The model under review builds one solid part; all positions refer to its coordinate system, in mm. Face numbers are marked on the shaded views. A direction names the side the tool comes from. Coordinates: 2 decimals unless noted, no trailing zeros. Order: outer loops, then holes, each group sorted by start corner. A loop starts at its lowest first (then second) coordinate and runs counter-clockwise, first axis right, second up. Notation, with made-up numbers: (84.5, -30) - (140.5, -30) arc R19 cw to (140.5, -9) - close; hole circle Ø2 at (-29, -39.5). An arc over 180 degrees is marked (long way). Answer in a Markdown table with one row per item.
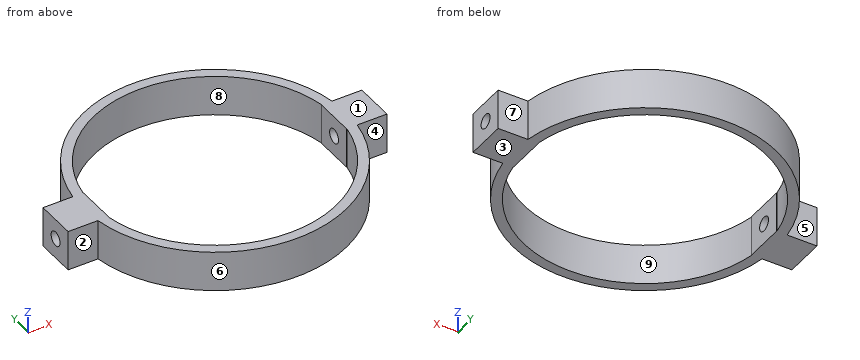
```python
from build123d import *

# Parameters (mm, degrees)
F0_R     = 41.275
F0_R_2   = 38.1
F1_DEPTH = 12.7
F3_W     = 12.7
F3_H     = 12.7
F4_DEPTH = 12.7
F6_W     = 12.7
F6_H     = 12.7
F7_DEPTH = 12.7
F9_D     = 4.4958


with BuildPart() as f1:
    # F0 (on Top) → F1 (new body)
    with BuildSketch(Plane.XY):
        Circle(F0_R)
        Circle(F0_R_2, mode=Mode.SUBTRACT)
    extrude(amount=F1_DEPTH)

    # F3 (on offset) → F4 (join)
    with BuildSketch(Plane.YZ.offset(37.465)):
        with Locations((0, 6.35)):
            Rectangle(F3_W, F3_H)
    extrude(amount=F4_DEPTH)

    # F6 (on offset) → F7 (join)
    with BuildSketch(Plane.YZ.offset(-37.465)):
        with Locations((0, 6.35)):
            Rectangle(F6_W, F6_H)
    extrude(amount=-F7_DEPTH)

    # F9 (through all)
    with Locations(Plane(origin=(-50.165, 0, 0), x_dir=(0, -1, 0), z_dir=(-1, 0, 0))):
        with Locations((0, 6.35)):
            Hole(F9_D / 2)


solid = f1.part
```
Item 1: Tool access review of the marked faces 1, 2, 3, 4 and 5: name each direction out of +Z, -Z, +X, -X, +Y, -Y from which nothing blocks a thin tool from reaching the whole face with its end or side.
Check values:
| item | result |
|---|---|
| face 1 | +Z, +X, -X, +Y, -Y |
| face 2 | +Z, -Z, -X, -Y |
| face 3 | -Z, +X, -X, +Y, -Y |
| face 4 | +Z, -Z, +X, -Y |
| face 5 | +Z, -Z, -X, +Y |
Item 2: We need section C-C, the plane x = 42. Write out the cut boundary in (y, z), then the cut area to 3 significant figures.
Check values:
| item | result |
|---|---|
| outline | (-6.35, 0) - (6.35, 0) - (6.35, 12.7) - (-6.35, 12.7) - close; hole circle Ø4.5 at (0, 6.35) |
| area | 145 mm^2 |
Item 3: To check wall thickness, follow line 1 (Z direction, x = 40.5, y = 0); line 2 (X direction, y = 5.5, z = 3) (3 decimals); line 3 (X direction, y = -32.5, z = 1.5). State the ranges of each line that lie inside material, in increasing order. Write a range as from..to.
Check values:
| item | result |
|---|---|
| line 1 | 0..4.1, 8.6..12.7 |
| line 2 | -50.165..-37.465, 37.465..50.165 |
| line 3 | -25.44..-19.88, 19.88..25.44 |
Item 4: We need section D-D, the plane y = 22. Write out the cut boundary in (x, z).
Check values:
| item | result |
|---|---|
| outline | (-34.92, 0) - (-31.11, 0) - (-31.11, 12.7) - (-34.92, 12.7) - close; (31.11, 0) - (34.92, 0) - (34.92, 12.7) - (31.11, 12.7) - close |
Item 5: Clearance check with flat-ended pins moving along their axes: pin 1 Ø4.5 at (x, z) = (45.5, 4.5) entering from +Y; pin 2 Ø2 at (x, z) = (-30, 4.5) entering from -Y; pin 3 Ø4.5 at (x, z) = (-45, 3) entering from -Y; pin 4 Ø2.5 at (y, z) = (0, 6.35) entering from -X. State where each tip first meets the part, or that it passes through.
Check values:
| item | result |
|---|---|
| pin 1 | y = 6.35 |
| pin 2 | y = -29.37 |
| pin 3 | y = -6.35 |
| pin 4 | through |
Item 6: We need section A-A, the plane z = 6.35. Write out the cut boundary in (x, y) (3 decimals), then the cut area to 3 significant figures.
Check values:
| item | result |
|---|---|
| outline | (-50.165, -6.35) - (-40.784, -6.35) arc R41.275 ccw to (40.784, -6.35) - (50.165, -6.35) - (50.165, -2.248) - (37.465, -2.248) - (37.465, -6.35) - (37.567, -6.35) arc R38.1 cw to (-37.567, -6.35) - (-37.465, -6.35) - (-37.465, -2.248) - (-50.165, -2.248) - close; (-50.165, 2.248) - (-37.465, 2.248) - (-37.465, 6.35) - (-37.567, 6.35) arc R38.1 cw to (37.567, 6.35) - (37.465, 6.35) - (37.465, 2.248) - (50.165, 2.248) - (50.165, 6.35) - (40.784, 6.35) arc R41.275 ccw to (-40.784, 6.35) - (-50.165, 6.35) - close |
| area | 919 mm^2 |
Item 7: Mouldability with a two-part tool opening along X and no side actions: class the marked faces 6, 7, 8 and 9 as +X half, -X half, draft (parallel to the pull), parting line (faces both ways), or undercut.
Check values:
| item | result |
|---|---|
| face 6 | parting line |
| face 7 | draft |
| face 8 | undercut |
| face 9 | undercut |
Item 8: We need section B-B, the plane y = 0. Write out the cut boundary in (x, z) (3 decimals), then the cut area to 3 significant figures.
Check values:
| item | result |
|---|---|
| outline | (-50.165, 0) - (-37.465, 0) - (-37.465, 4.102) - (-50.165, 4.102) - close; (-50.165, 8.598) - (-37.465, 8.598) - (-37.465, 12.7) - (-50.165, 12.7) - close; (37.465, 0) - (50.165, 0) - (50.165, 4.102) - (37.465, 4.102) - close; (37.465, 8.598) - (50.165, 8.598) - (50.165, 12.7) - (37.465, 12.7) - close |
| area | 208 mm^2 |
